Could you check a few things on this model? Use its own coordinates, in mm. Face numbers are marked on the shaded views. A direction names the side the tool comes from. Round coordinates to 2 decimals unless told otherwise and drop trailing zeros. Loops run counter-clockwise (first coordinate to the right, second up) from the corner with the lowest first, then second, coordinate; pieces in that order, holes last.
from build123d import *

# Parameters (mm, degrees)
CUT_EXTRUDE1_DEPTH = 32.004


# Read off the part's stored shape, not the designer's step: 1/2-20 Machine Threads Stud1
with BuildPart() as part:
    # Sketch2 → Revolve1 (revolve)
    with BuildSketch(Plane.XY):
        Polygon((0, 0), (0, 23.241), (6.35, 23.241), (6.35, 10.033), (339.979, 10.033), (339.979, 0), align=None)
    revolve(axis=Axis((339.979, 0, 0), (-1, 0, 0)))

    # 1/2-20 Machine Threads Stud1 outline → 1/2-20 Machine Threads Stud1 (revolve, cut)
    with BuildSketch(Plane.YX):
        Polygon((10.033, 339.979), (5.59435, 339.979), (6.35, 339.22335), (6.35, 317.627), (10.033, 317.627), align=None)
    revolve(axis=Axis((0, 0, 0), (1, 0, 0)), mode=Mode.SUBTRACT)

    # Sketch7 → Cut-Extrude1 (cut)
    with BuildSketch(Plane(origin=(339.979, 0, 0), x_dir=(0, 0, -1), z_dir=(1, 0, 0))):
        with BuildLine():
            Line((-6.35, 7.767791771), (-6.35, -7.767791771))
            ThreePointArc((-6.35, -7.767791771), (-10.033, 0), (-6.35, 7.767791771))
        make_face()
        with BuildLine():
            Line((6.35, 7.767791771), (6.35, -7.767791771))
            ThreePointArc((6.35, -7.767791771), (10.033, 0), (6.35, 7.767791771))
        make_face()
    extrude(amount=-CUT_EXTRUDE1_DEPTH, mode=Mode.SUBTRACT)


solid = part.part
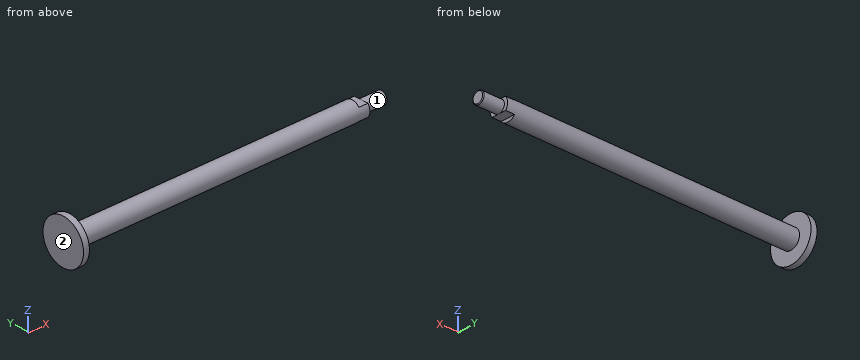
Item 1: If we section it at C-C, the plane y = 17: Please give me the cut outline in (x, z).
Results list:
outline: (0, -15.85) - (6.35, -15.85) - (6.35, 15.85) - (0, 15.85) - close
Item 2: For the marked faces 1 and 2, which set-ups out of +Z, -Z, +X, -X, +Y, -Y let a thin tool reach every point of the face, with its end or its side?
Results list:
face 1: +X
face 2: +Z, -Z, -X, +Y, -Y
Item 3: If we section it at A-A, the plane z = 0: Please give me the cut outline in (x, y), then the cut area to 3 significant figures.
Results list:
outline: (0, -23.24) - (6.35, -23.24) - (6.35, -10.03) - (317.63, -10.03) - (317.63, -6.35) - (339.22, -6.35) - (339.98, -5.59) - (339.98, 5.59) - (339.22, 6.35) - (317.63, 6.35) - (317.63, 10.03) - (6.35, 10.03) - (6.35, 23.24) - (0, 23.24) - close
area: 6,820 mm2
Item 4: If we section it at B-B, the plane x = 187: Please give me the cut outline in (y, z).
Results list:
outline: circle Ø20.07 at (0, 0)
Item 5: If we section it at D-D, the plane z = -13: Please give me the cut outline in (x, y).
Results list:
outline: (0, -19.27) - (6.35, -19.27) - (6.35, 19.27) - (0, 19.27) - close
Item 6: Will these pins go through, and if not, where does the flat tip stop? pin 1 (6 mm diameter, centred on y = 11, z = 8, fed in from +X); pin 2 (10.5 mm diameter, centred on x = 312, y = -4, fed in from -Z); pin 3 (7.5 mm diameter, centred on x = 312.5, y = -3, fed in from +Z); pin 4 (12 mm diameter, centred on x = 261.5, y = -17, fed in from +Z).
Results list:
pin 1: stops at x = 6.35
pin 2: stops at z = -10.01
pin 3: stops at z = 6.35
pin 4: passes through
Item 7: If I drill on line 1 along X through (y, z) = (14.5, 4.5); line 2 along X through (y, z) = (-5.5, -8) (3 decimals); line 3 along Z through (x, y) = (322, 3), over which ranges is the centre line in solid material (lowest first)?
Results list:
line 1: x = 0 to 6.35
line 2: x = 0 to 307.975
line 3: z = -5.6 to 5.6
